For this review, take the finished solid that the model builds, in its own axes (mm). Face numbers are marked on the shaded views. A direction names the side the tool comes from. Coordinates: 2 decimals unless noted, no trailing zeros. Order: outer loops, then holes, each group sorted by start corner. A loop starts at its lowest first (then second) coordinate and runs counter-clockwise, first axis right, second up.
Autodesk Fusion 360 part; units mm, degrees
sketch "Base" plane through (0, 0, 0) normal (0, 1, 0) x (1, 0, 0)
  line L0 (44, 33.5) -> (-44, 33.5)
  line L1 (44, -10.9853) -> (44, 33.5)
  line L2 (44, 33.5) -> (-44, -33.5) construction
  line L3 (-44, 33.5) -> (44, -33.5) construction
  line L4 (-44, 33.5) -> (44, 33.5)
  line L5 (44, 33.5) -> (44, 30.5)
  line L6 (-44, 30.5) -> (-44, 33.5)
  line L7 (-44, 30.5) -> (-40.0597, 30.5)
  line L8 (-44, -10.9853) -> (-44, 30.5)
  line L9 (44, -10.9853) -> (44, 30.5)
  arc A0 (-13.435, -46.935) -> (13.435, -46.935) centre (0, -33.5) ccw
  line L10 (0, -33.5) -> (-13.435, -46.935) construction
  line L11 (0, -33.5) -> (13.435, -46.935) construction
  line L12 (-13.435, -46.935) -> (-40.1924, -20.1777)
  line L13 (13.435, -46.935) -> (40.1924, -20.1777)
  line L14 (-44, 33.5) -> (-44, -10.9853)
  arc A1 (40.1924, -20.1777) -> (44, -10.9853) centre (31, -10.9853) ccw
  arc A2 (-44, -10.9853) -> (-40.1924, -20.1777) centre (-31, -10.9853) ccw
  line L15 (-44, 33.5) -> (44, 33.5)
  line L16 (44, 33.5) -> (44, 2.5)
  line L17 (-44, 2.5) -> (-44, 33.5)
  line L18 (0, 33.5) -> (-25, 33.5)
  line L19 (-25, -33.5) -> (0, -33.5) construction
  line L20 (0, -33.5) -> (25, -33.5) construction
  line L21 (25, 33.5) -> (0, 33.5)
  circle A3 centre (-25, 2.5) radius 5
  circle A4 centre (25, 2.5) radius 5
  line L22 (-44, 33.5) -> (44, 33.5)
  line L23 (44, 33.5) -> (44, 46.5)
  line L24 (-44, 46.5) -> (-44, 33.5)
  line L25 (-44, 46.5) -> (-25, 46.5)
  line L26 (-19, 33.5) -> (-44, 33.5)
  line L27 (-44, 33.5) -> (-44, 46.5)
  line L28 (44, 46.5) -> (25, 46.5)
  line L29 (19, 33.5) -> (44, 33.5)
  line L30 (44, 33.5) -> (44, 46.5)
  line L31 (44, 46.5) -> (44, 52.5) construction
  line L32 (44, 52.5) -> (-44, 52.5) construction
  line L33 (-44, 52.5) -> (-44, 46.5) construction
  circle A5 centre (0, 52.5) radius 9.5
  arc A6 (-25, 46.5) -> (-19, 52.5) centre (-25, 52.5) ccw
  arc A7 (19, 52.5) -> (25, 46.5) centre (25, 52.5) ccw
  arc A8 (19, 52.5) -> (-19, 52.5) centre (0, 52.5) ccw
  line L34 (-44, 46.5) -> (-25, 46.5)
  line L35 (25, 46.5) -> (44, 46.5)
  line L36 (44, 46.5) -> (25, 46.5)
  line L37 (-25, 46.5) -> (-44, 46.5)
  dimension "d1" = 88
  dimension "d2" = 67
  dimension "d3" = 3
  dimension "d6" = 38
  dimension "d10" = 13
  dimension "d11" = 31
  dimension "d12" = 25
  dimension "d13" = 25
  dimension "d14" = 10
  dimension "d15" = 10
  dimension "d38" = 13
  dimension "d43" = 6
  dimension "d44" = 19
  dimension "d45" = 38
  dimension "d46" = 6
  dimension "d47" = 6
extrude "Extrude1" add sketch "Base" along normal blind 10 contours L0 L1 L4 L5 L6 L8 L9 A0 L12 L13 L14 A1 A2 L15 L16 L17 L18 L21 L22 L26 L29
sketch "Base decorations" plane through (0, 10, 0) normal (0, 1, 0) x (-1, 0, 0)
  circle A0 centre (-25, -2.5) radius 5
  circle A1 centre (25, -2.5) radius 5
  line L0 (-44, -33.5) -> (44, -33.5)
  line L1 (44, -33.5) -> (44, 10.9853)
  arc A2 (44, 10.9853) -> (40.1924, 20.1777) centre (31, 10.9853) ccw
  line L2 (40.1924, 20.1777) -> (13.435, 46.935)
  arc A3 (13.435, 46.935) -> (-13.435, 46.935) centre (0, 33.5) ccw
  line L3 (-13.435, 46.935) -> (-40.1924, 20.1777)
  arc A4 (-40.1924, 20.1777) -> (-44, 10.9853) centre (-31, 10.9853) ccw
  line L4 (-44, 10.9853) -> (-44, -33.5)
  line L5 (44, -33.5) -> (-44, -33.5)
  line L6 (-44, -33.5) -> (-44, -30.5)
  line L7 (44, -30.5) -> (44, -33.5)
  line L8 (44, -30.5) -> (19, -30.5)
  line L9 (44, 10.5) -> (44, -30.5)
  line L10 (-44, -30.5) -> (-19, -30.5)
  line L11 (-44, 10.5) -> (-44, -30.5)
  line L12 (19, -30.5) -> (5, -30.5)
  line L13 (5, -30.5) -> (5, 10.5)
  line L14 (-19, -30.5) -> (-5, -30.5)
  line L15 (-5, -30.5) -> (-5, 10.5)
  line L16 (-5, -30.5) -> (-5, -26.5)
  line L17 (-5, -26.5) -> (5, -26.5)
  line L18 (5, -26.5) -> (5, -30.5)
  line L19 (5, -33.5) -> (-5, -33.5)
  line L20 (-5, -30.5) -> (-5, 33.5)
  line L21 (-5, 33.5) -> (5, 33.5)
  line L22 (5, 33.5) -> (5, -30.5)
  line L23 (-44, -30.5) -> (-5, -30.5)
  line L24 (5, -30.5) -> (44, -30.5)
  line L25 (19, -30.5) -> (5, -30.5)
  line L26 (-5, -30.5) -> (-19, -30.5)
  line L27 (44, -33.5) -> (19, -33.5)
  line L28 (19, -30.5) -> (44, -30.5)
  line L29 (44, -30.5) -> (44, -33.5)
  line L30 (-44, -33.5) -> (-19, -33.5)
  line L31 (-19, -30.5) -> (-44, -30.5)
  line L32 (-44, -30.5) -> (-44, -33.5)
  arc A5 (-22, -33.5) -> (-19, -30.5) centre (-22, -30.5) ccw
  arc A6 (19, -30.5) -> (22, -33.5) centre (22, -30.5) ccw
  dimension "d18" = 3
  dimension "d19" = 25
  dimension "d20" = 41
  dimension "d21" = 25
  dimension "d22" = 41
  dimension "d23" = 14
  dimension "d24" = 14
  dimension "d26" = 4
  dimension "d27" = 67
  dimension "d28" = 25
  dimension "d29" = 25
  dimension "d30" = 3
  dimension "d31" = 3
extrude "Extrude4" add sketch "Base decorations" along normal blind 40 contours L0 L5 L12 L13 L14 L15 L16 L17 L18 L19 L20 L22 L23 L24 L25 L26 L27 L30 A5 A6
extrude "Extrude2" add sketch "Base decorations" along normal blind 40 contours L13 L15 L17 L20 L21 L22
sketch "Triangle cut" plane through (5, 0, 0) normal (1, 0, 0) x (0, 0, -1)
  line L0 (-33.5, 10) -> (30.5, 10)
  line L1 (30.5, 50) -> (-33.5, 50)
  line L2 (-33.5, 50) -> (-33.5, 10)
  line L3 (30.5, 50) -> (-33.5, 10)
  line L4 (30.5, 10) -> (30.5, 50)
extrude "Extrude3" cut sketch "Triangle cut" against normal blind 10 contours L1 L2 L3
extrude "Extrude5" add sketch "Base" along normal blind 50 contours L0 L4 L15 L18 L21 L22 L23 L24 L25 L26 L27 L28 L29 L30 A6 A7 A8 L34 L35 L36 L37
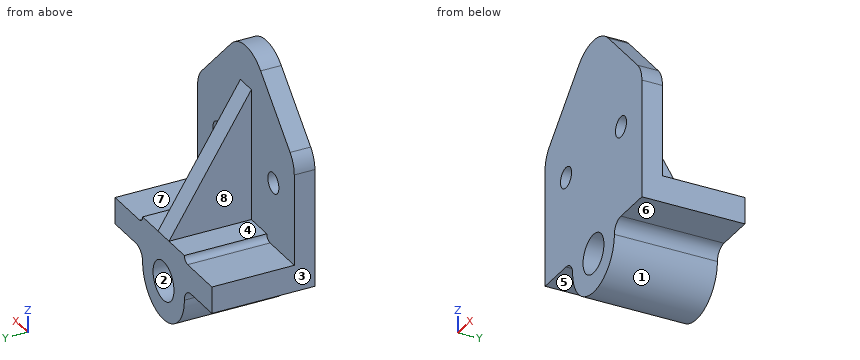
1. The part is to be moulded in two halves that separate along X. For the marked faces 1, 2, 3 and 4, say which applies: +X half, -X half, draft (parallel to the pull), parting line (faces both ways), or undercut.
Answer below:
face 1: parting line
face 2: undercut
face 3: -X half
face 4: draft
2. Machinability: for the marked faces 5, 6, 7 and 8, which of the approach directions +Z, -Z, +X, -X, +Y, -Y give a long, thin tool a straight path to every point of the face, cutting with its end or side? Answer none if there is none.
Answer below:
face 5: -Z, -X, +Y, -Y
face 6: -Z, +X, +Y, -Y
face 7: +Z, +X, +Y
face 8: +Z, -X, +Y
3. Take a section at A-A, the plane z = -2.5. Give the boundary of the cut face in (x, y), plus the area to 3 significant figures.
Answer below:
outline: (-44, 0) - (-30, 0) - (-30, 10) - (-44, 10) - close; (-20, 0) - (20, 0) - (20, 10) - (5, 10) - (5, 32.5) - (-5, 32.5) - (-5, 10) - (-20, 10) - close; (30, 0) - (44, 0) - (44, 10) - (30, 10) - close
area: 905 mm2
4. Take a section at B-B, the plane y = 4. Give the boundary of the cut face in (x, z) (3 decimals), plus the area to 3 significant figures.
Answer below:
outline: (-44, -46.5) - (-25, -46.5) arc R6 cw to (-19, -52.5) arc R19 ccw to (19, -52.5) arc R6 cw to (25, -46.5) - (44, -46.5) - (44, 10.985) arc R13 ccw to (40.192, 20.178) - (13.435, 46.935) arc R19 ccw to (-13.435, 46.935) - (-40.192, 20.178) arc R13 ccw to (-44, 10.985) - close; hole circle Ø10 at (-25, -2.5); hole circle Ø19 at (0, -52.5); hole circle Ø10 at (25, -2.5)
area: 7,750 mm2
5. Take a section at C-C, the plane x = 0. Give the boundary of the cut face in (y, z), plus the area to 3 significant figures.
Answer below:
outline: (0, -71.5) - (50, -71.5) - (50, -62) - (0, -62) - close; (0, -43) - (50, -43) - (50, -30.5) - (10, 33.5) - (10, 52.5) - (0, 52.5) - close
area: 3,210 mm2
6. Clearance check with flat-ended pins moving along their axes: pin 1 Ø12 at (y, z) = (30.5, -13.5) entering from +X; pin 2 Ø24 at (x, y) = (-36, 36) entering from +Z; pin 3 Ø11 at (x, y) = (-13.5, 29) entering from +Z. State where each tip first meets the part, or that it passes through.
Answer below:
pin 1: stops at x = 5
pin 2: stops at z = -33.5
pin 3: stops at z = -30.5
7. Take a section at D-D, the plane y = 13. Give the boundary of the cut face in (x, z), plus the area to 3 significant figures.
Answer below:
outline: (-44, -46.5) - (-25, -46.5) arc R6 cw to (-19, -52.5) arc R19 ccw to (19, -52.5) arc R6 cw to (25, -46.5) - (44, -46.5) - (44, -33.5) - (22, -33.5) arc R3 cw to (19, -30.5) - (5, -30.5) - (5, 28.7) - (-5, 28.7) - (-5, -30.5) - (-19, -30.5) arc R3 cw to (-22, -33.5) - (-44, -33.5) - close; hole circle Ø19 at (0, -52.5)
area: 2,380 mm2
8. To check wall thickness, follow L1, parallel to X at y = 7, z = -2; L2, parallel to X at y = 16.5, z = -52.5; L3, parallel to Z at x = -39, y = 15. State the ranges of each line that lie inside material, in increasing order.
Answer below:
L1: x = -44 to -29.97, -20.03 to 20.03, 29.97 to 44
L2: x = -19 to -9.5, 9.5 to 19
L3: z = -46.5 to -33.5
